```python
from build123d import *

# Parameters (mm, degrees)
F0_R      = 2.5
F1_DEPTH  = 45
F2_R      = 7.9375
F2_R_2    = 12.7
F3_DEPTH  = 114.301
F5_DEPTH  = 35
F7_DEPTH  = 114.301
F8_SIZE   = 10
F9_R      = 8.15
F10_DEPTH = 25
F10_TAPER = 5.72
F13_R     = 0.5
F14_DEPTH = 2000


with BuildPart() as f1:
    # F0 (on Front) → F1 (new body)
    with BuildSketch(Plane.XZ):
        with BuildLine():
            Line((0, 40), (0, 0))
            Line((0, 0), (114.3, 0))
            Line((114.3, 0), (114.3, 120))
            Line((114.3, 120), (49.3399335472, 322.0957796647))
            ThreePointArc((49.3399335472, 322.0957796647), (27.4308241539, 336.8342969493), (10, 317))
            Line((10, 317), (10, 237))
            Line((10, 237), (15, 120))
            Line((15, 120), (15, 50))
            ThreePointArc((15, 50), (12.0710678119, 42.9289321881), (5, 40))
            Line((5, 40), (0, 40))
        make_face()
        with BuildLine():
            ThreePointArc((57.15, 130), (64.2210678119, 127.0710678119), (67.15, 120))
            Line((67.15, 120), (67.15, 60))
            ThreePointArc((67.15, 60), (64.2210678119, 52.9289321881), (57.15, 50))
            ThreePointArc((57.15, 50), (50.0789321881, 52.9289321881), (47.15, 60))
            Line((47.15, 60), (47.15, 120))
            ThreePointArc((47.15, 120), (50.0789321881, 127.0710678119), (57.15, 130))
        make_face(mode=Mode.SUBTRACT)
        with Locations((30, 317)):
            Circle(F0_R, mode=Mode.SUBTRACT)
    extrude(amount=F1_DEPTH)

    # F2 (on face) → F3 (cut, through all)
    with BuildSketch(Plane.YZ.offset(114.3)):
        with Locations((-25.5, 97.5)):
            Circle(F2_R)
        with Locations((-22.5, 20)):
            Circle(F2_R_2)
    extrude(amount=-F3_DEPTH, mode=Mode.SUBTRACT)

    # F4 (on face) → F5 (cut)
    with BuildSketch(Plane(origin=(0, 0, 0), x_dir=(-1, 0, 0), z_dir=(0, 1, 0))):
        with BuildLine():
            Line((-48.4216344216, 253.0601220633), (-80.5648422415, 153.0601220633))
            ThreePointArc((-80.5648422415, 153.0601220633), (-79.1254456583, 144.1093812139), (-71.0445663549, 140))
            Line((-71.0445663549, 140), (-45.7471559309, 140))
            ThreePointArc((-45.7471559309, 140), (-38.828688156, 142.7795565477), (-35.7562748619, 149.5730392706))
            Line((-35.7562748619, 149.5730392706), (-31.4827705884, 249.5730392706))
            ThreePointArc((-31.4827705884, 249.5730392706), (-33.8223810432, 256.438793209), (-40.1875050962, 259.9169464566))
            ThreePointArc((-40.1875050962, 259.9169464566), (-45.300475796, 257.6844842559), (-48.4216344216, 253.0601220633))
        make_face()
    extrude(amount=-F5_DEPTH, mode=Mode.SUBTRACT)

    # F6 (on face) → F7 (cut, through all)
    with BuildSketch(Plane(origin=(0, 0, 0), x_dir=(0, -1, 0), z_dir=(-1, 0, 0))):
        Polygon((75.7247351185, 458.4947787785), (22, 458.4947787785), (22, 291.8342969493), (75.7247351185, 198.7803261009), align=None)
    extrude(amount=-F7_DEPTH, mode=Mode.SUBTRACT)

    # F8
    f8_edges = [f1.edges().sort_by_distance(p)[0] for p in [
        (57.15, 0, 0),
        (57.15, -45, 0),
    ]]
    chamfer(f8_edges, length=F8_SIZE)

    # F9 (on face) → F10 (cut)
    with BuildSketch(Plane.XZ.offset(22)):
        with Locations((30, 317)):
            Circle(F9_R)
    extrude(amount=-F10_DEPTH, taper=F10_TAPER, mode=Mode.SUBTRACT)

    # F13 (on line) → F14 (join)
    with BuildSketch(Plane(origin=(0, -15.8124107275, 335.3013597184), x_dir=(1, 0, 0), z_dir=(0, -0.0471064507, 0.998889875))):
        with Locations((0, -20.920984447)):
            Circle(F13_R)
    extrude(amount=-F14_DEPTH)


solid = f1.part
```
Geometry check sheet. Reference: the model listing, model coordinates, mm. A direction names the side the tool comes from. Coordinates: 2 decimals unless noted, no trailing zeros. One line per item, written item: value. Start each with the question number.
(1) Mould release check, pull along Z, two halves, no side actions. Record for faces 1 (the flat face through (12.465, -22.185, 179.319)), 2 (the flat face through (82.275, -22.185, 219.633)), 3 (the flat face through (114.3, -22, 59)): released by +Z, released by -Z, zero draft, split by the parting line, or undercut.
(2) Tool access check on faces 4 (the flat face through (47.15, -22, 90)), 5 (the flat face through (33.65, -17.26, 198.87)), 6 (the flat face through (34.2, -22, 309.7)). Record the directions out of +Z, -Z, +X, -X, +Y, -Y that give a thin tool (end or side, any length) a straight path to the whole face; none if there is none.
(3) Material ranges on line 1 (Z direction, x = 27.5, y = -22.5); line 2 (Y direction, x = 83, z = 20); line 3 (Z direction, x = 39, y = -32.5), recorded low to high. Write a range as [from, to].
(4) Depth check by flat-ended pin: P1, Ø6, axis at y = 37.5, z = -1363, coming from the -X side; P2, Ø2.5, axis at x = 1.5, y = -15, coming from the +Z side; P3, Ø22.5, axis at y = -29.5, z = 101.5, coming from the -X side; P4, Ø12.5, axis at y = -25.5, z = 97.5, coming from the +X side. Enter the tip coordinate at first touch or a pass-through.
Results below:
1. face 1: undercut
1. face 2: released by +Z
1. face 3: zero draft
2. face 4: +Y, -Y
2. face 5: +Y
2. face 6: +Z, +X, -X, -Y
3. line 1: z = [0, 7.3], [32.7, 90.15], [104.85, 290.97]
3. line 2: y = [-45, -35.2], [-9.8, 0]
3. line 3: z = [0, 12.17], [27.83, 93.76], [101.24, 142.62], [259.69, 273.65]
4. P1: passes through
4. P2: stops at z = 40
4. P3: stops at x = -0.5
4. P4: stops at x = 0.5
